Check sheet for the modelled part. Datum: model origin and axes. Units: mm. Face numbers are marked on the shaded views. Round coordinates to 2 decimals unless told otherwise and drop trailing zeros.
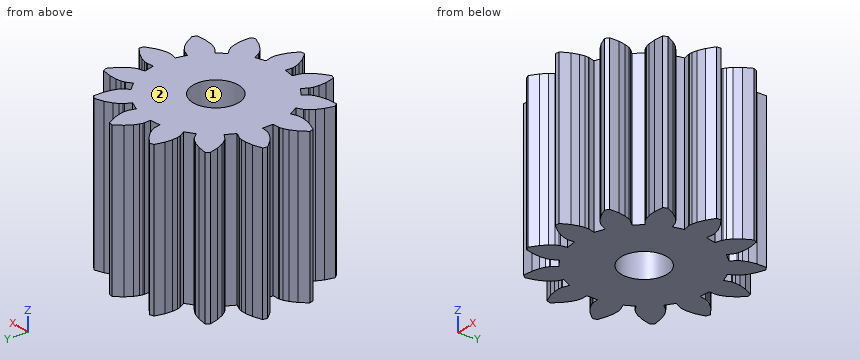
from build123d import *

# Parameters (mm, degrees)
CYLINDER001_R          = 1.5
CYLINDER001_DEPTH      = 12
LINEAREXTRUDE001_DEPTH = 10


with BuildPart() as cylinder001:
    # cylinder001 → cylinder001 (new body)
    with BuildSketch(Plane.XY.offset(-1)):
        Circle(CYLINDER001_R)
    extrude(amount=CYLINDER001_DEPTH)


with BuildPart() as difference002:
    # union001 → LinearExtrude001 (new body)
    with BuildSketch(Plane(origin=(0, 0, 0), x_dir=(0, 1, 0), z_dir=(0, 0, 1))):
        Polygon((0.711931, -4.306123), (1.370771, -4.143733), (1.502069, -4.540636), (1.530367, -4.602072), (1.641751, -4.771632), (1.871155, -5.020002), (2.245545, -5.309618), (2.782207, -5.596589), (3.025427, -5.468937), (3.094113, -4.864255), (3.068442, -4.391617), (2.994354, -4.061731), (2.918082, -3.873743), (2.883597, -3.815555), (2.631538, -3.482032), (3.139447, -3.032064), (3.440155, -3.322487), (3.493763, -3.363735), (3.671187, -3.46211), (3.989737, -3.575421), (4.455834, -3.657875), (5.064387, -3.662577), (5.220426, -3.436516), (5.000234, -2.869177), (4.757857, -2.462607), (4.53895, -2.204938), (4.384052, -2.073928), (4.326475, -2.038431), (3.948292, -1.860249), (4.188912, -1.225786), (4.590143, -1.343197), (4.656779, -1.354807), (4.859597, -1.359461), (5.194318, -1.311756), (5.645345, -1.168159), (6.186377, -0.889514), (6.219486, -0.616832), (5.76086, -0.216806), (5.357304, 0.030555), (5.043726, 0.156979), (4.845688, 0.200998), (4.77821, 0.205671), (4.36054, 0.187693), (4.278749, 0.861305), (4.688584, 0.943805), (4.752983, 0.964491), (4.934732, 1.054624), (5.208943, 1.252418), (5.541575, 1.58917), (5.891142, 2.087328), (5.793738, 2.344162), (5.201743, 2.485233), (4.729457, 2.516719), (4.393046, 2.482935), (4.197235, 2.429879), (4.135314, 2.402658), (3.773841, 2.192639), (3.388376, 2.751081), (3.712928, 3.01459), (3.760337, 3.062835), (3.879381, 3.227107), (4.030263, 3.529677), (4.168298, 3.982437), (4.246318, 4.585986), (4.040715, 4.768136), (3.45097, 4.617935), (3.018149, 4.426332), (2.735972, 4.240079), (2.587247, 4.102103), (2.545069, 4.049224), (2.322601, 3.695276), (1.721767, 4.010618), (1.886685, 4.394771), (1.906243, 4.459522), (1.93531, 4.6603), (1.928298, 4.99833), (1.840114, 5.463378), (1.628715, 6.034052), (1.362012, 6.099788), (0.909622, 5.692724), (0.61542, 5.321926), (0.452121, 5.025874), (0.384552, 4.834585), (0.371779, 4.768162), (0.339281, 4.351371), (-0.339281, 4.351371), (-0.371779, 4.768162), (-0.384552, 4.834585), (-0.452121, 5.025874), (-0.61542, 5.321926), (-0.909622, 5.692724), (-1.362012, 6.099788), (-1.628715, 6.034052), (-1.840114, 5.463378), (-1.928298, 4.99833), (-1.93531, 4.6603), (-1.906243, 4.459522), (-1.886685, 4.394771), (-1.721767, 4.010618), (-2.322601, 3.695276), (-2.545069, 4.049224), (-2.587247, 4.102103), (-2.735972, 4.240079), (-3.018149, 4.426332), (-3.45097, 4.617935), (-4.040715, 4.768136), (-4.246318, 4.585986), (-4.168298, 3.982437), (-4.030263, 3.529677), (-3.879381, 3.227107), (-3.760337, 3.062835), (-3.712928, 3.01459), (-3.388376, 2.751081), (-3.773841, 2.192638), (-4.135314, 2.402658), (-4.197235, 2.429879), (-4.393046, 2.482935), (-4.729457, 2.516719), (-5.201743, 2.485233), (-5.793738, 2.344162), (-5.891142, 2.087328), (-5.541575, 1.58917), (-5.208943, 1.252418), (-4.934732, 1.054624), (-4.752983, 0.964491), (-4.688584, 0.943805), (-4.278749, 0.861305), (-4.36054, 0.187693), (-4.77821, 0.205671), (-4.845688, 0.200998), (-5.043726, 0.156979), (-5.357304, 0.030555), (-5.76086, -0.216806), (-6.219486, -0.616832), (-6.186377, -0.889514), (-5.645345, -1.168159), (-5.194318, -1.311756), (-4.859597, -1.359461), (-4.656779, -1.354807), (-4.590143, -1.343197), (-4.188912, -1.225786), (-3.948292, -1.860249), (-4.326475, -2.038431), (-4.384052, -2.073928), (-4.53895, -2.204938), (-4.757857, -2.462607), (-5.000234, -2.869177), (-5.220426, -3.436516), (-5.064387, -3.662577), (-4.455834, -3.657875), (-3.989737, -3.575421), (-3.671187, -3.46211), (-3.493763, -3.363735), (-3.440155, -3.322487), (-3.139447, -3.032064), (-2.631537, -3.482032), (-2.883597, -3.815555), (-2.918082, -3.873743), (-2.994354, -4.061731), (-3.068442, -4.391617), (-3.094113, -4.864255), (-3.025427, -5.468937), (-2.782207, -5.596589), (-2.245545, -5.309618), (-1.871155, -5.020002), (-1.641751, -4.771632), (-1.530367, -4.602072), (-1.502069, -4.540636), (-1.370771, -4.143733), (-0.71193, -4.306122), (-0.780122, -4.71858), (-0.783616, -4.78613), (-0.763789, -4.98803), (-0.676085, -5.31456), (-0.47917, -5.74499), (-0.137342, -6.24849), (0.137342, -6.24849), (0.47917, -5.74499), (0.676085, -5.31456), (0.763789, -4.98803), (0.783616, -4.78613), (0.780122, -4.71858), align=None)
    extrude(amount=LINEAREXTRUDE001_DEPTH)

    # difference002: cut cylinder001
    add(cylinder001.part, mode=Mode.SUBTRACT)


with BuildPart() as difference002_1:
    # difference002 placement: moved
    add(difference002.part.moved(Location((11, 0, 0))))


solid = difference002_1.part
1) Draft check along X on the marked faces 1 and 2. Enter one of: pulls with the +X half, pulls with the -X half, needs draft (parallel to the pull), parting line crosses it, or undercut.
2) Gauge pin test, flat end, axial feed: pin 1 (1.5 mm diameter, centred on x = 10, z = 1.5, fed in from -Y). Record the tip position at first contact, or that the pin passes through.
3) Scan lines: line 1 (X direction, y = 0, z = 4); line 2 (X direction, y = 4.75, z = 3.5); line 3 (Y direction, x = 12.75, z = 1.5). Record each from-to range of solid material in increasing order.
Values found:
1. face 1: undercut
1. face 2: needs draft
2. pin 1: stops at y = -5.65
3. line 1: x = 6.65 to 9.5, 12.5 to 17.25
3. line 2: x = 8.48 to 10.04, 10.8 to 12.36, 13.45 to 14.66
3. line 3: y = -3.99 to 3.99
